Verification items for the finished model (mm, model axes). Face numbers are marked on the shaded views. A direction names the side the tool comes from. Give positions to 0.01 mm unless a question says otherwise; leave off trailing zeros. Write each loop counter-clockwise with the first axis right and the second up, starting at its lowest first coordinate (ties: lowest second). Pieces come first, ordered by that corner, then holes. Notation, with made-up numbers: (48, 15) -> (89, 15) arc R19 cw to (89, 34) -> close; hole circle Ø5 at (20, 6.25). An arc over 180 degrees is marked (long way). Write item = value, one per line.
from build123d import *

# Parameters (mm, degrees)
F0_R     = 3.175
F1_DEPTH = 63.5
F2_W     = 60.96
F2_H     = 21.8726252659
F3_DEPTH = 152.401


with BuildPart() as f1:
    # F0 (on Front) → F1 (new body)
    with BuildSketch(Plane.XZ):
        with BuildLine():
            Line((70.2170193255, -6.4695058077), (-69.4829806745, -6.4695058077))
            ThreePointArc((-69.4829806745, -6.4695058077), (-73.973108735, -8.3293777471), (-75.8329806745, -12.8195058077))
            Line((-75.8329806745, -12.8195058077), (-75.8329806745, -19.1695058077))
            Line((-75.8329806745, -19.1695058077), (76.5670193255, -19.1695058077))
            Line((76.5670193255, -19.1695058077), (76.5670193255, -12.8195058077))
            ThreePointArc((76.5670193255, -12.8195058077), (74.707147386, -8.3293777471), (70.2170193255, -6.4695058077))
        make_face()
        with Locations((-69.4829806745, -12.8195058077)):
            Circle(F0_R, mode=Mode.SUBTRACT)
        with Locations((70.2170193255, -12.8195058077)):
            Circle(F0_R, mode=Mode.SUBTRACT)
    extrude(amount=F1_DEPTH)

    # F2 (on face) → F3 (cut, through all)
    with BuildSketch(Plane(origin=(-75.8329806745, 0, 0), x_dir=(0, -1, 0), z_dir=(-1, 0, 0))):
        with Locations((31.75, -1.8831931747)):
            Rectangle(F2_W, F2_H)
        with BuildLine():
            Line((62.23, -12.8195058077), (1.27, -12.8195058077))
            Line((1.27, -12.8195058077), (1.27, -17.2645058077))
            ThreePointArc((1.27, -17.2645058077), (1.4559871939, -17.7135186137), (1.905, -17.8995058077))
            Line((1.905, -17.8995058077), (61.595, -17.8995058077))
            ThreePointArc((61.595, -17.8995058077), (62.0440128061, -17.7135186137), (62.23, -17.2645058077))
            Line((62.23, -17.2645058077), (62.23, -12.8195058077))
        make_face()
    extrude(amount=-F3_DEPTH, mode=Mode.SUBTRACT)


solid = f1.part
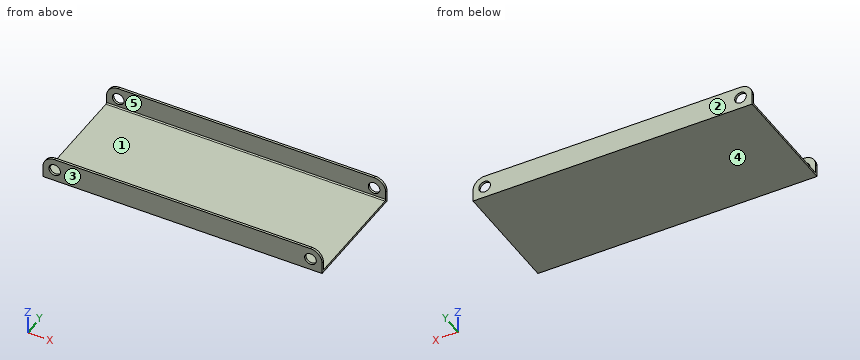
Item 1: Sectioned sample at A-A on z = -14.25. Record the cut outline in (x, y).
Response values:
outline = (-75.83, -63.5) -> (-72.32, -63.5) -> (-72.32, -62.23) -> (-75.83, -62.23) -> close; (-75.83, -1.27) -> (-72.32, -1.27) -> (-72.32, 0) -> (-75.83, 0) -> close; (-66.65, -63.5) -> (67.38, -63.5) -> (67.38, -62.23) -> (-66.65, -62.23) -> close; (-66.65, -1.27) -> (67.38, -1.27) -> (67.38, 0) -> (-66.65, 0) -> close; (73.05, -63.5) -> (76.57, -63.5) -> (76.57, -62.23) -> (73.05, -62.23) -> close; (73.05, -1.27) -> (76.57, -1.27) -> (76.57, 0) -> (73.05, 0) -> close
Item 2: Go/stop test with a flat-tipped pin: P1, Ø1, axis at x = -22, y = -29, coming from the +Z side. Record where the tip stops, or that it passes through.
Response values:
P1 = -17.9
Item 3: Set-up check for the marked faces 4 and 5: record each of +Z, -Z, +X, -X, +Y, -Y from which the full face is reachable in a straight line by a thin tool's end or side.
Response values:
face_4 = -Z, +X, -X, +Y, -Y
face_5 = +Z, +X, -X
Item 4: Sectioned sample at B-B on x = 22. Record the cut outline in (y, z) (1 decimal), then the cut area to 3 significant figures.
Response values:
outline = (-63.5, -19.2) -> (0, -19.2) -> (0, -6.5) -> (-1.3, -6.5) -> (-1.3, -17.3) arc R0.6 cw to (-1.9, -17.9) -> (-61.6, -17.9) arc R0.6 cw to (-62.2, -17.3) -> (-62.2, -6.5) -> (-63.5, -6.5) -> close
area = 110 mm^2
Item 5: Material ranges on line 1 (Y direction, x = -13, z = -11.25); line 2 (Z direction, x = -4, y = -53), recorded low to high.
Response values:
line_1 = -63.5 to -62.23, -1.27 to 0
line_2 = -19.17 to -17.9
Item 6: Mould release check, pull along Y, two halves, no side actions. Record for the marked faces 1, 2 and 3: +Y half, -Y half, draft (parallel to the pull), parting line (faces both ways), or undercut.
Response values:
face_1 = undercut
face_2 = +Y half
face_3 = -Y half
Item 7: Sectioned sample at C-C on y = -49. Record the cut outline in (x, z).
Response values:
outline = (-75.83, -19.17) -> (76.57, -19.17) -> (76.57, -17.9) -> (-75.83, -17.9) -> close
